Read the model definition and answer for the solid it produces. Units are mm, in the model's axes. A direction names the side the tool comes from. Round coordinates to 2 decimals unless told otherwise and drop trailing zeros. Order: outer loops, then holes, each group sorted by start corner. A loop starts at its lowest first (then second) coordinate and runs counter-clockwise, first axis right, second up. Notation, with made-up numbers: (40, 13.25) - (88, 13.25) arc R19 cw to (88, 31.25) - close; hole circle Ø1 at (8.5, 23.5). An arc over 180 degrees is marked (long way). One line per question, with ' | ' between items. Start each with the question number.
1) For faces 4 (the cylindrical face through (5.388, 17.406, 1.479)), 5 (the flat face through (12, 12, 0)), determine the directions among +Z, -Z, +X, -X, +Y, -Y from which every point of the face is accessible in a straight line to the end or side of a thin tool.
2) The part is cut by section C-C, the plane x = 20. Give the vertices of the cut face in (y, z), plus the area to 3 significant figures.
3) The part is cut by section A-A, the plane x = 4.1. Give the vertices of the cut face in (y, z), plus the area to 3 significant figures.
4) Straight lines are drawn through the part: line 1 (Y direction, x = 20.1, z = 2.45); line 2 (Y direction, x = 4.1, z = 1.2); line 3 (X direction, y = 16, z = 2.5). For each, find the intervals that lie inside material, in ascending order. Write a range as from..to.
5) The mould has two halves that part along Y. Classify faces 1 (the cylindrical face through (0.301, 0.285, 1.521)), 2 (the flat face through (12, 12, 3)), 3 (the cylindrical face through (30.22, 6.44, -4.31)): pulls with the +Y half, pulls with the -Y half, needs draft (parallel to the pull), parting line crosses it, or undercut.
6) Flat-ended cylindrical pins translate along their axes: pin 1 (2 mm diameter, centred on x = 20.1, y = 15, fed in from -Z); pin 2 (1 mm diameter, centred on x = 10.5, y = 3.5, fed in from -Z); pin 3 (1.5 mm diameter, centred on x = 24, y = 8, fed in from -Z); pin 4 (3 mm diameter, centred on y = 16.5, z = -4.5, fed in from -X). Find the tip coordinate at first contact, or state that the pin passes through.
7) The part is cut by section D-D, the plane y = 21.5. Give the vertices of the cut face in (x, z).
8) The part is cut by section B-B, the plane y = 15. Give the vertices of the cut face in (x, z), plus the area to 3 significant figures.
from build123d import *

# Parameters (mm, degrees)
SKETCH_W     = 25
SKETCH_H     = 24
SKETCH_R     = 1.35
PAD_DEPTH    = 3
PAD001_DEPTH = 24
SKETCH002_R  = 1.6
POCKET_DEPTH = 26.67867
FILLET_R     = 1


with BuildPart() as part:
    # Sketch → Pad (new body)
    with BuildSketch(Plane.XY):
        with Locations((12.5, 12)):
            Rectangle(SKETCH_W, SKETCH_H)
        with Locations((4.1, 17)):
            Circle(SKETCH_R, mode=Mode.SUBTRACT)
        with Locations((20.1, 15)):
            Circle(SKETCH_R, mode=Mode.SUBTRACT)
        with Locations((4.1, 7)):
            Circle(SKETCH_R, mode=Mode.SUBTRACT)
        with Locations((20.1, 7)):
            Circle(SKETCH_R, mode=Mode.SUBTRACT)
    extrude(amount=PAD_DEPTH)

    # Sketch001 (on Face3 of Pad) → Pad001 (join)
    with BuildSketch(Plane(origin=(0, 24, 0), x_dir=(-1, 0, 0), z_dir=(0, 1, 0))):
        Polygon((-25, 3), (-35.606602, -7.606602), (-33.485281, -9.727922), (-22.87868, 0.87868), align=None)
    extrude(amount=-PAD001_DEPTH)

    # Sketch002 (on Face13 of Pad001) → Pocket (cut, through all)
    with BuildSketch(Plane(origin=(14, 0, 14), x_dir=(0, 1, 0), z_dir=(0.707107, 0, 0.707107))):
        with Locations((5.7, -23)):
            Circle(SKETCH002_R)
        with Locations((18.2, -23)):
            Circle(SKETCH002_R)
    extrude(amount=-POCKET_DEPTH, mode=Mode.SUBTRACT)

    # Fillet
    fillet_edges = [part.edges().sort_by_distance(p)[0] for p in [
        (34.545942, 24, -8.667262),
        (34.545942, 0, -8.667262),
        (0, 24, 1.5),
        (0, 0, 1.5),
    ]]
    fillet(fillet_edges, radius=FILLET_R)


solid = part.part
Values:
1) face 4: +Z, -Z | face 5: -Z, -X, +Y, -Y
2) outline: (0, 0) - (5.65, 0) - (5.65, 3) - (0, 3) - close; (8.35, 0) - (13.65, 0) - (13.65, 3) - (8.35, 3) - close; (16.35, 0) - (24, 0) - (24, 3) - (16.35, 3) - close | area: 55.8 mm^2
3) outline: (0, 0) - (5.65, 0) - (5.65, 3) - (0, 3) - close; (8.35, 0) - (15.65, 0) - (15.65, 3) - (8.35, 3) - close; (18.35, 0) - (24, 0) - (24, 3) - (18.35, 3) - close | area: 55.8 mm^2
4) line 1: y = 0..5.65, 8.35..13.65, 16.35..24 | line 2: y = 0..5.65, 8.35..15.65, 18.35..24 | line 3: x = 0..3.19, 5.01..19.19, 21.01..25.5
5) face 1: pulls with the -Y half | face 2: needs draft | face 3: undercut
6) pin 1: passes through | pin 2: stops at z = 0 | pin 3: stops at z = -0.99 | pin 4: stops at x = 26.76
7) outline: (0, 0) - (23.76, 0) - (33.49, -9.73) - (35.61, -7.61) - (25, 3) - (0, 3) - close
8) outline: (0, 0) - (18.75, 0) - (18.75, 3) - (0, 3) - close; (21.45, 0) - (23.76, 0) - (33.49, -9.73) - (35.61, -7.61) - (25, 3) - (21.45, 3) - close | area: 108 mm^2
